Part model, mm, in its own coordinate system. Face numbers are marked on the shaded views. A direction names the side the tool comes from. Give positions to 0.01 mm unless a question says otherwise; leave off trailing zeros. Order: outer loops, then holes, each group sorted by start corner. A loop starts at its lowest first (then second) coordinate and runs counter-clockwise, first axis right, second up. Notation, with made-up numbers: (37, 39.25) - (58, 39.25) arc R19 cw to (58, 43.25) - close; hole circle Ø8 at (68.5, -17.75). An arc over 180 degrees is marked (long way). One line per item, written item: value.
```python
from build123d import *

# Parameters (mm, degrees)
SKETCH1_R           = 3.37312
SKETCH1_R_2         = 2.33426
BOSS_EXTRUDE1_DEPTH = 4.2545
SKETCH2_R           = 0.4699
BOSS_EXTRUDE2_DEPTH = 1.2192
SKETCH3_R           = 2.33426
BOSS_EXTRUDE3_DEPTH = 1.5621
SKETCH4_R           = 1.9685
BOSS_EXTRUDE5_DEPTH = 5.1308


with BuildPart() as part:
    # Sketch1 → Boss-Extrude1 (new body)
    with BuildSketch(Plane.XY):
        Circle(SKETCH1_R)
        Circle(SKETCH1_R_2, mode=Mode.SUBTRACT)
    extrude(amount=BOSS_EXTRUDE1_DEPTH)

    # Sketch2 → Boss-Extrude2 (add)
    with BuildSketch(Plane.XY.offset(4.2545)):
        with BuildLine():
            ThreePointArc((1.87014753, 5.114443216), (0, 6.4685), (-1.87014753, 5.114443216))
            Line((-1.87014753, 5.114443216), (-3.204588284, 1.052878181))
            ThreePointArc((-3.204588284, 1.052878181), (0, 3.37312), (3.204588284, 1.052878181))
            Line((3.204588284, 1.052878181), (1.87014753, 5.114443216))
        make_face()
        with Locations((0, 4.5)):
            Circle(SKETCH2_R, mode=Mode.SUBTRACT)
    extrude(amount=-BOSS_EXTRUDE2_DEPTH)

    # Sketch3 → Boss-Extrude3 (add)
    with BuildSketch(Plane.XY.offset(4.2545)):
        Circle(SKETCH3_R)
    extrude(amount=-BOSS_EXTRUDE3_DEPTH)

    # Sketch4 → Boss-Extrude5 (add)
    with BuildSketch(Plane.XY.offset(4.2545)):
        with Locations((0, 4.5)):
            Circle(SKETCH4_R)
    extrude(amount=BOSS_EXTRUDE5_DEPTH)


solid = part.part
```
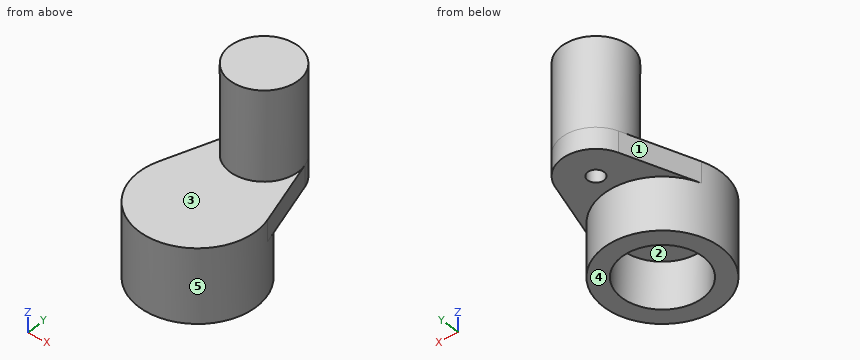
1) Slice it at D-D on y = 4.5. Write the cut outline in (x, z), then the cut area to 3 significant figures.
Answer:
outline: (-2.07, 3.04) - (-0.47, 3.04) - (-0.47, 4.25) - (0.47, 4.25) - (0.47, 3.04) - (2.07, 3.04) - (2.07, 4.25) - (1.97, 4.25) - (1.97, 9.39) - (-1.97, 9.39) - (-1.97, 4.25) - (-2.07, 4.25) - close
area: 24.1 mm2
2) Slice it at B-B on y = 2. Write the cut outline in (x, z), then the cut area to 3 significant figures.
Answer:
outline: (-2.89, 3.04) - (-2.72, 3.04) - (-2.72, 0) - (-1.2, 0) - (-1.2, 2.69) - (1.2, 2.69) - (1.2, 0) - (2.72, 0) - (2.72, 3.04) - (2.89, 3.04) - (2.89, 4.25) - (-2.89, 4.25) - close
area: 17.1 mm2
3) Wall check: line 1 along Y through (x, z) = (0, 1.1); line 2 along Z through (x, y) = (-1, 5.5); line 3 along Z through (x, y) = (-1.5, -1). Give the ranges that are in metal, low to high. Write a range as [from, to].
Answer:
line 1: y = [-3.37, -2.33], [2.33, 3.37]
line 2: z = [3.04, 9.39]
line 3: z = [2.69, 4.25]
4) Two-plate mould, pull along X, no slides. Class the marked faces 1, 2 and 3: pulls with the +X half, pulls with the -X half, needs draft (parallel to the pull), parting line crosses it, or undercut.
Answer:
face 1: pulls with the -X half
face 2: undercut
face 3: needs draft
5) Slice it at A-A on x = 0. Write the cut outline in (y, z), then the cut area to 3 significant figures.
Answer:
outline: (-3.37, 0) - (-2.33, 0) - (-2.33, 2.69) - (2.33, 2.69) - (2.33, 0) - (3.37, 0) - (3.37, 3.04) - (4.03, 3.04) - (4.03, 4.25) - (4.97, 4.25) - (4.97, 3.04) - (6.47, 3.04) - (6.47, 9.39) - (2.53, 9.39) - (2.53, 4.25) - (-3.37, 4.25) - close
area: 39.0 mm2
6) Which spindle directions (+Z, -Z, +X, -X, +Y, -Y) get a long thin tool onto all of the face, cutting with end or side? Do the marked faces 4 and 5. Say none if no direction does.
Answer:
face 4: -Z, +X, -X, +Y, -Y
face 5: -Z
7) Slice it at C-C on z = 7. Write the cut outline in (x, y), then the cut area to 3 significant figures.
Answer:
outline: circle Ø3.94 at (0, 4.5)
area: 12.2 mm2
8) Drop flat-ended pins along their axis: P1, Ø2, axis at y = 2.5, z = 6.5, coming from the -X side; P2, Ø1.5, axis at x = -1.5, z = 3.5, coming from the +Y side; P3, Ø0.5, axis at x = 0, y = 4.5, coming from the -Z side. Give the stop position or say it passes through.
Answer:
P1: stops at x = -1.7
P2: stops at y = 6.32
P3: stops at z = 4.25
